```python
from build123d import *

# Parameters (mm, degrees)
F0_W     = 330.2
F0_H     = 38.1
F2_DEPTH = 12.7
F1_R     = 12.7
F1_R_2   = 6.35
F3_DEPTH = 12.7


with BuildPart() as f2:
    # F0 (on Top) → F2 (new body, symmetric)
    with BuildSketch(Plane.XY):
        with Locations((1.8771, 2.322538)):
            Rectangle(F0_W, F0_H)
    extrude(amount=F2_DEPTH, both=True)

    # F1 (on Top) → F3 (cut, symmetric)
    with BuildSketch(Plane.XY):
        with Locations((-135.067344, 0)):
            Circle(F1_R)
        with Locations((133.833691, 0)):
            Circle(F1_R_2)
    extrude(amount=F3_DEPTH, both=True, mode=Mode.SUBTRACT)


solid = f2.part
```
Input: part model. Units: mm. Frame: model coordinates. Coordinates: 2 decimals unless noted, no trailing zeros. Order: outer loops, then holes, each group sorted by start corner. A loop starts at its lowest first (then second) coordinate and runs counter-clockwise, first axis right, second up. Notation, with made-up numbers: (66.25, 74.25) - (101.25, 74.25) arc R19 ccw to (101.25, 109.25) - close; hole circle Ø9 at (-24, -23). An arc over 180 degrees is marked (long way). Put each result on its own line as item: value.
1. Cut plane A-A on y = 0. Return the cut outline in (x, z).
Report:
outline: (-163.22, -12.7) - (-147.77, -12.7) - (-147.77, 12.7) - (-163.22, 12.7) - close; (-122.37, -12.7) - (127.48, -12.7) - (127.48, 12.7) - (-122.37, 12.7) - close; (140.18, -12.7) - (166.98, -12.7) - (166.98, 12.7) - (140.18, 12.7) - close
2. Draft query along X for faces 1 (the face through (0, -16.727, 0)), 2 (the face through (-163.223, 2, 0)), 3 (the face through (139.89, 1.91, 0.18)). Return one class per face: pulls with the +X half, pulls with the -X half, needs draft (parallel to the pull), parting line crosses it, or undercut.
Report:
face 1: needs draft
face 2: pulls with the -X half
face 3: undercut
3. Line query: line 1 along X through (y, z) = (4.5, -0.5); line 2 along X through (y, z) = (4, -0.75); line 3 along X through (y, z) = (-8, 4). Output: solid intervals per line, ascending.
Report:
line 1: x = -163.22 to -146.94, -123.19 to 129.35, 138.31 to 166.98
line 2: x = -163.22 to -147.12, -123.01 to 128.9, 138.77 to 166.98
line 3: x = -163.22 to -144.93, -125.2 to 166.98
4. Cut plane B-B on z = 5.25. Return the cut outline in (x, y).
Report:
outline: (-163.22, -16.73) - (166.98, -16.73) - (166.98, 21.37) - (-163.22, 21.37) - close; hole circle Ø25.4 at (-135.07, 0); hole circle Ø12.7 at (133.83, 0)
5. Contact query for a flat-ended pin moving along its axis: pin 1 Ø10 at (x, y) = (133.83, 0) entering from -Z. Output: stop coordinate, or through.
Report:
pin 1: passes through
